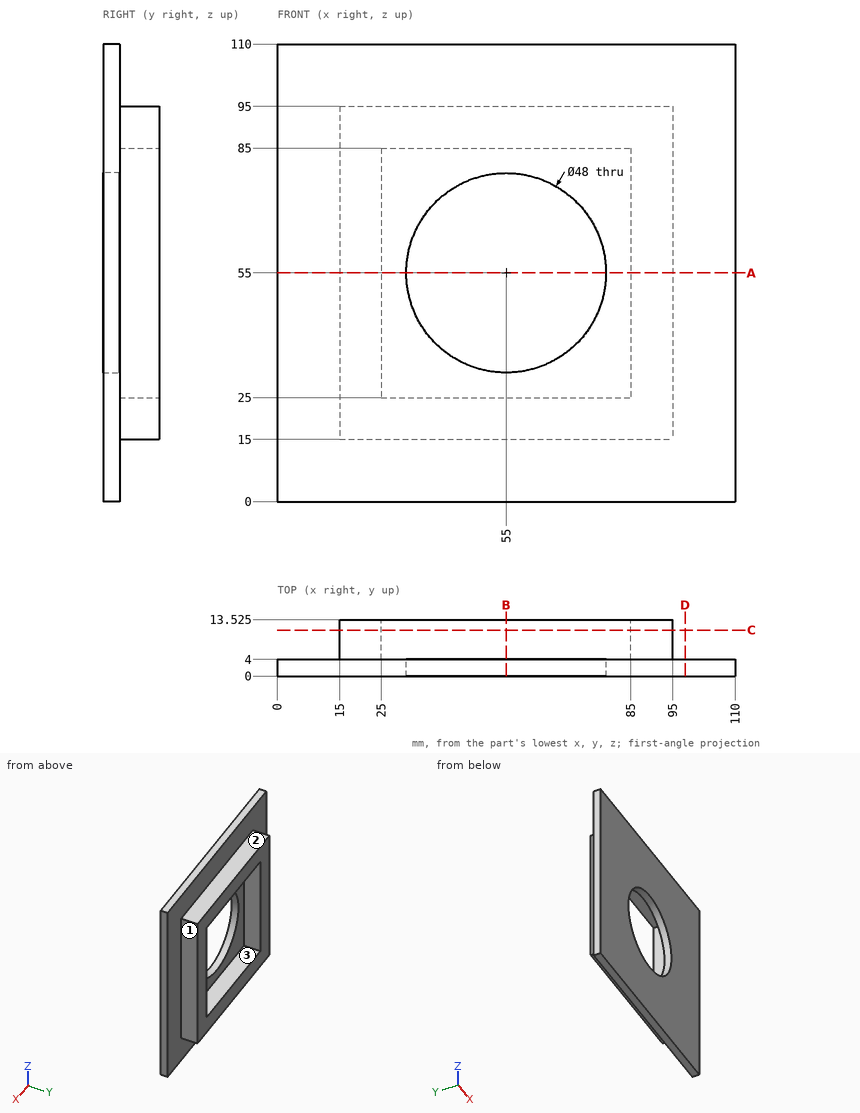
The figure shows three views and two pictorial views of one solid part (mm, origin at its lowest corner). Answer the questions. A direction names the side the tool comes from. Give positions to 0.01 mm unless a question says otherwise; leave off trailing zeros. Write each loop counter-clockwise with the first axis right and the second up, starting at its lowest first coordinate (ties: lowest second). Pieces come first, ordered by that corner, then holes. Notation, with made-up numbers: M -17.75,79 L 38.25,79 A34 ccw 38.25,111 Z; hole C 61,-32 d7. An arc over 180 degrees is marked long. One line per item, written item: value. Start each with the question number.
(1) Find section C-C (y = 11). Determine the outline of the cut face in (x, z), plus the area to 3 significant figures.
(2) A tool of negligible diameter and unlimited length cuts with its end or side. For the marked faces 1, 2 and 3, from which of +Z, -Z, +X, -X, +Y, -Y can it reach the whole face along a straight path? Write none if from no direction.
(3) Flat-ended cylindrical pins translate along their axes: pin 1 Ø3 at (y, z) = (8, 62) entering from +X; pin 2 Ø3 at (y, z) = (11, 62) entering from -X; pin 3 Ø5 at (x, y) = (51.5, 7) entering from +Z. Find the tip coordinate at first contact, or state that the pin passes through.
(4) Find the intervals of material crossed by line 1 (X direction, y = 11.5, z = 60.5); line 2 (X direction, y = 2.9, z = 55), in increasing order.
(5) Find section A-A (z = 55). Determine the outline of the cut face in (x, y) (3 decimals).
(6) Find section B-B (x = 55). Determine the outline of the cut face in (y, z) (3 decimals).
(7) Find section D-D (x = 98). Determine the outline of the cut face in (y, z), plus the area to 3 significant figures.
Results below:
1. outline: M 15,15 L 95,15 L 95,95 L 15,95 Z; hole M 25,25 L 85,25 L 85,85 L 25,85 Z
1. area: 2,800 mm^2
2. face 1: +Z, -Z, +X, +Y
2. face 2: +Z, +X, -X, +Y
2. face 3: +Y
3. pin 1: stops at x = 95
3. pin 2: stops at x = 15
3. pin 3: stops at z = 95
4. line 1: x = 15 to 25, 85 to 95
4. line 2: x = 0 to 31, 79 to 110
5. outline: M 0,0 L 31,0 L 31,4 L 25,4 L 25,13.525 L 15,13.525 L 15,4 L 0,4 Z; M 79,0 L 110,0 L 110,4 L 95,4 L 95,13.525 L 85,13.525 L 85,4 L 79,4 Z
6. outline: M 0,0 L 4,0 L 4,15 L 13.525,15 L 13.525,25 L 4,25 L 4,31 L 0,31 Z; M 0,79 L 4,79 L 4,85 L 13.525,85 L 13.525,95 L 4,95 L 4,110 L 0,110 Z
7. outline: M 0,0 L 4,0 L 4,110 L 0,110 Z
7. area: 440 mm^2
